Geometry: final body of the model. Coordinates: model frame, mm. A direction names the side the tool comes from. Round coordinates to 2 decimals unless told otherwise and drop trailing zeros. Loops run counter-clockwise (first coordinate to the right, second up) from the corner with the lowest first, then second, coordinate; pieces in that order, holes last. Notation, with made-up numbers: (28.5, 12.25) - (45.5, 12.25) arc R18 cw to (45.5, 38.25) - close; hole circle Ø11 at (-6.75, 88.25). An arc over 180 degrees is marked (long way). Return JSON: item names as keys, results as strings. Group by question number.
1. First-contact query: pin 1 Ø4 at (x, y) = (0.5, -20) entering from +Z; pin 2 Ø5 at (x, y) = (-3.5, -17.5) entering from -Z; pin 3 Ø4 at (y, z) = (-49.5, -1) entering from -X. Flat tips, straight axial feed; report the tip coordinate or a pass-through.
2. Section B-B on y = -7. Return loops of the section in (x, z), and give its area (3 significant figures).
3. Set-up query: faces 1 (the face through (4, -24.45, 2)), 2 (the face through (3.3, -3.45, -0.1)), 3 (the face through (0, -55.1, 0)). Return all of +Z, -Z, +X, -X, +Y, -Y with unobstructed straight access to the full face (end or side cutting, diameter ignored); none if empty.
4. Section A-A on y = -25.5. Return loops of the section in (x, z).
5. Material intervals for probe 1 along Z at (x, y) = (4, -8.5); probe 2 along Y at (x, z) = (-3, 3.5), sorted ascending.
Autodesk Inventor part; units mm, degrees
ref_plane "YZ Plane" through (0, 0, 0) normal (1, 0, 0) x (0, 1, 0)
ref_plane "XZ Plane" through (0, 0, 0) normal (0, 1, 0) x (-1, 0, 0)
ref_plane "XY Plane" through (0, 0, 0) normal (0, 0, 1) x (1, 0, 0)
sketch "Sketch1" plane through (0, 0, 0) normal (0, 1, 0) x (-1, 0, 0)
  circle A0 centre (0, 0) radius 2.5
  circle A1 centre (0, 0) radius 3
  line L0 (0, 2.5) -> (0, -2.5)
  dimension "d0" = 5
  dimension "d1" = 6
extrude "Extrusion1" add sketch "Sketch1" against normal blind 15 contours A0 L0 | L0 A0 | A1
revolve "Revolution1" cut sketch "Sketch1" angle 360 about axis through (0, 0, 2.5) along (0, 0, -1) picked at (0.5196, 0.6515) contours A0 L0
sketch "Sketch2" plane through (0, 0, 0) normal (0, 1, 0) x (1, 0, 0)
  circle A0 centre (0, 0) radius 3
  circle A1 centre (0, 0) radius 2.5
extrude "Extrusion2" cut sketch "Sketch2" against normal blind 1.1 contours A0 | A1
sketch "Sketch3" plane through (0, -15, 0) normal (0, -1, 0) x (1, 0, 0)
  circle A0 centre (0, 0) radius 5
  circle A1 centre (0, 0) radius 3
  dimension "d7" = 10
extrude "Extrusion3" add sketch "Sketch3" against normal blind 10
sketch "Sketch4" plane through (0, -15, 0) normal (0, -1, 0) x (1, 0, 0)
  circle A0 centre (0, 0) radius 5
extrude "Extrusion4" cut sketch "Sketch4" against normal blind 5
sketch "Sketch5" plane through (0, -10, 0) normal (0, -1, 0) x (1, 0, 0)
  circle A0 centre (0, 0) radius 3.95
  dimension "d12" = 7.9
extrude "Extrusion5" add sketch "Sketch5" along normal blind 45
sketch "Sketch6" plane through (0, -5, 0) normal (0, 1, 0) x (1, 0, 0)
  circle A0 centre (0, 0) radius 3
  circle A1 centre (0, 0) radius 5
extrude "Extrusion6" cut sketch "Sketch6" against normal blind 0.1
sketch "Sketch7" plane through (0, -10, 0) normal (0, -1, 0) x (1, 0, 0)
  circle A0 centre (0, 0) radius 5
  circle A1 centre (0, 0) radius 3.95
extrude "Extrusion7" add sketch "Sketch7" along normal blind 0.1
sketch "Sketch8" plane through (0, -55, 0) normal (0, -1, 0) x (1, 0, 0)
  circle A0 centre (0, 0) radius 3.95
extrude "Extrusion8" add sketch "Sketch8" along normal blind 0.1
sketch "Sketch9" plane through (0, -5.1, 0) normal (0, 1, 0) x (1, 0, 0)
  circle A0 centre (0, 0) radius 5
extrude "Extrusion9" add sketch "Sketch9" along normal blind 2
sketch "Sketch10" plane through (0, -10.1, 0) normal (0, -1, 0) x (1, 0, 0)
  circle A0 centre (0, 0) radius 5
  circle A1 centre (0, 0) radius 3.95
extrude "Extrusion10" cut sketch "Sketch10" against normal blind 2
extrude "Extrusion11" add sketch "Sketch10" against normal blind 2
extrude "Extrusion12" add sketch "Sketch10" along normal blind 14.7
sketch "Sketch11" plane through (0, -1.1, 0) normal (0, 1, 0) x (1, 0, 0)
  circle A0 centre (0, 0) radius 3
extrude "Extrusion13" cut sketch "Sketch11" against normal blind 0.3
sketch "Sketch12" plane through (0, -3.1, 0) normal (0, 1, 0) x (1, 0, 0)
  circle A0 centre (0, 0) radius 5
  circle A1 centre (0, 0) radius 3
extrude "Extrusion14" cut sketch "Sketch12" against normal blind 0.35
sketch "Sketch13" plane through (0, -24.8, 0) normal (0, -1, 0) x (1, 0, 0)
  circle A0 centre (0, 0) radius 3.95
  circle A1 centre (0, 0) radius 5
extrude "Extrusion15" cut sketch "Sketch13" against normal blind 0.35
sketch "Sketch14" plane through (0, -1.4, 0) normal (0, 1, 0) x (1, 0, 0)
  circle A0 centre (0, 0) radius 2.0712
  circle A1 centre (0, 0) radius 3
extrude "Extrusion16" cut sketch "Sketch14" against normal blind 0.2 contours A0 | A1
fillet "Fillet1" radius 2 1 edges at (-3.95, -55.1, 0)
properties part number "BARRA V3_3DPrint"
Taken from the geometry:
{
 "1": {"pin 1": "z = 5", "pin 2": "z = -4.9", "pin 3": "x = -3.95"},
 "2": {"outline": "circle Ø10 at (0, 0)", "area": "78.5 mm2"},
 "3": {"face 1": "-Y", "face 2": "+Y", "face 3": "+Z, -Z, +X, -X, -Y"},
 "4": {"outline": "circle Ø7.9 at (0, 0)"},
 "5": {"probe 1": "-3 to 3", "probe 2": "-24.45 to -3.45"}
}
